Build history of the part. All positions in model axes, mm. A direction names the side the tool comes from. Round coordinates to 2 decimals unless told otherwise and drop trailing zeros. Write each loop counter-clockwise with the first axis right and the second up, starting at its lowest first coordinate (ties: lowest second). Pieces come first, ordered by that corner, then holes. Notation, with made-up numbers: M 37.25,82.25 L 42.25,82.25 A26 cw 42.25,113.25 Z; hole C -14,12 d3. An arc over 180 degrees is marked long. Write item = value, one per line. Start each with the question number.
Q1. Probe L1, parallel to X at y = 14, z = 4.5; L2, parallel to Y at x = -9.25, z = 1.75; L3, parallel to Y at x = -3, z = 4. List the from-to ranges inside material, lowest first.
Q2. Band-saw the part on C-C on x = -3.5. Write the cut outline in (y, z), plus the area to 3 significant figures.
Q3. Pull direction Y, two halves, no side cores. Call faces 6 (the flat face through (-9, 3.8, 8)), 7 (the cylindrical face through (-11.6, 1.9, 5.5)), 8 (the cylindrical face through (-2.74, 10.4, 2.69)): released by +Y, released by -Y, zero draft, split by the parting line, or undercut.
Q4. Tool access for faces 1 (the cylindrical face through (-0.862, 15.115, 0.301)), 2 (the cylindrical face through (-2.27, 2.3, 5.63)), 3 (the cylindrical face through (-10.4, 2.74, 2.69)), 4 (the flat face through (-3.8, 9, 8)), 5 (the flat face through (0, 7, 6)): list every direction of +Z, -Z, +X, -X, +Y, -Y with a clear straight run to the whole face (end or side of a thin tool).
Q5. Band-saw the part on D-D on x = -9.5. Write the cut outline in (y, z).
Q6. Band-saw the part on A-A on z = 5.55. Write the cut outline in (x, y), plus the area to 4 significant figures.
Q7. Band-saw the part on B-B on y = 2.25. Write the cut outline in (x, z), plus the area to 3 significant figures.
Q8. Drop flat-ended pins along their axis: P1, Ø2, axis at y = 4, z = 8.5, coming from the -X side; P2, Ø3.5, axis at y = 9.5, z = 5.55, coming from the +X side; P3, Ø3.5, axis at y = 10.5, z = 5, coming from the -X side; P4, Ø5, axis at x = -8, z = 4.5, coming from the +Y side. Give the stop position or say it passes through.
```python
from build123d import *

# Parameters (mm, degrees)
EXTRUDE_1_DEPTH    = 11.1
FILLET_1_R         = 1
SKETCH_3_R         = 3
EXTRUDE_2_DEPTH    = 3.8
SKETCH_2_R         = 3
EXTRUDE_3_DEPTH    = 3.8
FILLET_2_R         = 2
HOLE_WIZARD_M5_3_D = 4.2
HOLE_WIZARD_M5_4_D = 4.2


with BuildPart() as part:
    # 草图1 → 凸台-拉伸1 (new body)
    with BuildSketch(Plane.XY):
        Polygon((0, 0), (0, 15.4), (-1.7, 15.4), (-1.7, 1.7), (-15.4, 1.7), (-15.4, 0), align=None)
    extrude(amount=EXTRUDE_1_DEPTH)

    # 圆角1
    fillet_1_edges = [part.edges().sort_by_distance(p)[0] for p in [
        (-0.85, 15.4, 11.1),
        (-15.4, 0.85, 11.1),
        (-15.4, 0.85, 0),
        (-0.85, 15.4, 0),
    ]]
    fillet(fillet_1_edges, radius=FILLET_1_R)

    # 草图3 → 凸台-拉伸2 (add)
    with BuildSketch(Plane(origin=(0, 0, 0), x_dir=(1, 0, 0), z_dir=(0, 1, 0))):
        with Locations(Location((-9.5, -5.55, 0), (0, 0, 90))):
            Circle(SKETCH_3_R)
    extrude(amount=EXTRUDE_2_DEPTH)

    # 草图2 → 凸台-拉伸3 (add)
    with BuildSketch(Plane(origin=(0, 0, 0), x_dir=(0, 0, -1), z_dir=(1, 0, 0))):
        with Locations((-5.55, 9.5)):
            Circle(SKETCH_2_R)
    extrude(amount=-EXTRUDE_3_DEPTH)

    # 圆角2
    fillet_2_edges = [part.edges().sort_by_distance(p)[0] for p in [
        (-1.7, 1.7, 5.55),
        (0, 0, 5.55),
    ]]
    fillet(fillet_2_edges, radius=FILLET_2_R)

    # M5 螺纹孔3 (through all)
    with Locations(Plane(origin=(0, 0, 0), x_dir=(0, 0, -1), z_dir=(1, 0, 0))):
        with Locations((-5.55, 9.5)):
            Hole(HOLE_WIZARD_M5_3_D / 2)

    # M5 螺纹孔4 (through all)
    with Locations(Plane(origin=(0, 0, 0), x_dir=(-1, 0, 0), z_dir=(0, -1, 0))):
        with Locations((9.5, -5.55)):
            Hole(HOLE_WIZARD_M5_4_D / 2)


solid = part.part
```
Conclusion:
q1.L1 = -1.7 to 0
q1.L2 = 0 to 1.7
q1.L3 = 0 to 1.83, 6.93 to 8.08, 10.92 to 12.07
q2.outline = M 0,0 L 1.71,0 L 1.71,11.1 L 0,11.1 Z; C 9.5,5.55 d6; hole C 9.5,5.55 d4.2
q2.area = 33.4 mm^2
q3.face_6 = released by +Y
q3.face_7 = zero draft
q3.face_8 = undercut
q4.face_1 = -Z, +X, -X, +Y
q4.face_2 = +Z, -Z
q4.face_3 = +Y
q4.face_4 = +Z, -Z, -X, +Y
q4.face_5 = +Z, -Z, +X, +Y, -Y
q5.outline = M 0,0 L 1.7,0 L 1.7,2.55 L 3.8,2.55 L 3.8,3.45 L 0,3.45 Z; M 0,7.65 L 3.8,7.65 L 3.8,8.55 L 1.7,8.55 L 1.7,11.1 L 0,11.1 Z
q6.outline = M -15.4,0 L -11.6,0 L -11.6,3.8 L -12.5,3.8 L -12.5,1.7 L -15.4,1.7 Z; M -7.4,0 L -2,0 A2 ccw 0,2 L 0,7.4 L -3.8,7.4 L -3.8,6.5 L -1.7,6.5 L -1.7,3.7 A2 cw -3.7,1.7 L -6.5,1.7 L -6.5,3.8 L -7.4,3.8 Z; M -3.8,11.6 L 0,11.6 L 0,15.4 L -1.7,15.4 L -1.7,12.5 L -3.8,12.5 Z
q6.area = 42.75 mm^2
q7.outline = C -9.5,5.55 d6; M -2.32,0 L 0,0 L 0,11.1 L -2.32,11.1 Z; hole C -9.5,5.55 d4.2
q7.area = 40.2 mm^2
q8.P1 = -11.76
q8.P2 = through
q8.P3 = -3.8
q8.P4 = 3.8
